Work out the finished part from the listing and answer in its coordinate system (mm). A direction names the side the tool comes from. Round coordinates to 2 decimals unless told otherwise and drop trailing zeros. Write each loop counter-clockwise with the first axis right and the second up, starting at its lowest first coordinate (ties: lowest second). Pieces come first, ordered by that corner, then holes.
1. Straight lines are drawn through the part: probe 1 along Z at (x, y) = (47, -35.5); probe 2 along Y at (x, z) = (64.5, 29.5). For each, find the intervals that lie inside material, in ascending order.
2. Find section B-B (y = -33). Write down the section's boundary in (x, z), and give its area (3 significant figures).
3. Flat-ended cylindrical pins translate along their axes: pin 1 Ø8 at (x, z) = (71, 25.5) entering from -Y; pin 2 Ø12 at (y, z) = (-45.5, 30) entering from +X; pin 3 Ø5 at (x, y) = (31, -27) entering from -Z; pin 4 Ø10 at (y, z) = (-42, 15.5) entering from +X. Find the tip coordinate at first contact, or state that the pin passes through.
4. Find section D-D (y = -47.5). Write down the section's boundary in (x, z), and give its area (3 significant figures).
5. A tool of negligible diameter and unlimited length cuts with its end or side. For faces 1 (the face through (0, -23, 20)), 2 (the face through (60, -10, 40)), 3 (the face through (31, -35, 20)), from which of +Z, -Z, +X, -X, +Y, -Y can it reach the whole face along a straight path? Write none if from no direction.
6. Find section A-A (x = 58). Write down the section's boundary in (y, z), and give its area (3 significant figures).
7. Find section C-C (z = 8). Write down the section's boundary in (x, y), and give its area (3 significant figures).
```python
from build123d import *

# Parameters (mm, degrees)
F1_DEPTH = 20
F2_W     = 40
F2_H     = 20
F3_DEPTH = 30
F4_DEPTH = 20
F6_DEPTH = 20


with BuildPart() as f1:
    # F0 (on Top) → F1 (new body)
    with BuildSketch(Plane.XY):
        Polygon((80, 0), (0, 0), (0, -60), (80, -20), align=None)
    extrude(amount=F1_DEPTH)

    # F2 (on face) → F3 (join)
    with BuildSketch(Plane.XY.offset(20)):
        with Locations((20, -10)):
            Rectangle(F2_W, F2_H)
    extrude(amount=F3_DEPTH)

    # F2 (on face) → F4 (join)
    with BuildSketch(Plane.XY.offset(20)):
        with Locations((60, -10)):
            Rectangle(F2_W, F2_H)
    extrude(amount=F4_DEPTH)

    # F5 (on face) → F6 (join)
    with BuildSketch(Plane(origin=(0, 0, 0), x_dir=(0, -1, 0), z_dir=(-1, 0, 0))):
        Polygon((40, 20), (20, 50), (20, 20), align=None)
    extrude(amount=-F6_DEPTH)


solid = f1.part
```
Worked answers:
1. probe 1: z = 0 to 20
1. probe 2: y = -20 to 0
2. outline: (0, 0) - (54, 0) - (54, 20) - (20, 20) - (20, 30.5) - (0, 30.5) - close
2. area: 1,290 mm2
3. pin 1: stops at y = -20
3. pin 2: passes through
3. pin 3: stops at z = 0
3. pin 4: stops at x = 46
4. outline: (0, 0) - (25, 0) - (25, 20) - (0, 20) - close
4. area: 500 mm2
5. face 1: +Z, -Z, -X, +Y, -Y
5. face 2: +Z, +X, +Y, -Y
5. face 3: +Z, +X, -Y
6. outline: (-31, 0) - (0, 0) - (0, 40) - (-20, 40) - (-20, 20) - (-31, 20) - close
6. area: 1,020 mm2
7. outline: (0, -60) - (80, -20) - (80, 0) - (0, 0) - close
7. area: 3,200 mm2
